The model under review builds one solid part; all positions refer to its coordinate system, in mm. A direction names the side the tool comes from. Round coordinates to 2 decimals unless told otherwise and drop trailing zeros. Loops run counter-clockwise (first coordinate to the right, second up) from the corner with the lowest first, then second, coordinate; pieces in that order, holes last. Notation, with made-up numbers: (57.25, 25.5) -> (70.25, 25.5) arc R28 ccw to (70.25, 48.5) -> close; hole circle Ø7 at (-20.75, 57.25). An arc over 180 degrees is marked (long way). Write each question's results on one line, items separated by ' | '. Start each with the question number.
Item 1: We need section D-D (x = -5). Give the boundary of the cut face in (y, z), and give its area (3 significant figures).
Item 2: Clearance check with flat-ended pins moving along their axes: pin 1 Ø7 at (x, z) = (-5, 11) entering from +Y; pin 2 Ø10.5 at (x, z) = (5, 17) entering from +Y; pin 3 Ø2.5 at (x, z) = (7, 29.5) entering from +Y. State where each tip first meets the part, or that it passes through.
Item 3: We need section C-C (x = 4.5). Give the boundary of the cut face in (y, z).
Item 4: We need section A-A (y = -15). Give the boundary of the cut face in (x, z), and give its area (3 significant figures).
Item 5: Tool access review of faces 4 (the cylindrical face through (-6.7, -21.5, 21.9)), 5 (the flat face through (0, -20.5, 22)), 6 (the flat face through (0, 25.5, 13)), 7 (the cylindrical face through (6.87, 21.49, 30.49)), 8 (the flat face through (0, -25.5, 13)): name each direction out of +Z, -Z, +X, -X, +Y, -Y from which nothing blocks a thin tool from reaching the whole face with its end or side.
Item 6: For L1, parallel to Y at x = 19, z = 3; L2, parallel to Y at x = -16.5, z = 31.5; L3, parallel to X at y = -22, z = 22, list the stretches that pass through material, from the lowest coordinate up. Write a range as from..to.
Item 7: We need section B-B (x = 19). Give the boundary of the cut face in (y, z), and give its area (3 significant figures).
Item 8: Mouldability with a two-part tool opening along X and no side actions: class faces 1 (the flat face through (-12, -21, 40)), 2 (the cylindrical face through (0.12, -21.51, 36.96)), 3 (the cylindrical face through (20.985, -21.514, 32.414)) as pulls with the +X half, pulls with the -X half, needs draft (parallel to the pull), parting line crosses it, or undercut.
from build123d import *

# Parameters (mm, degrees)
SKETCH_1_W          = 46
SKETCH_1_H          = 40
SKETCH_1_R          = 1.5
EXTRUDE_1_DEPTH     = 5
SKETCH_2_W          = 46
SKETCH_2_H          = 7.5
EXTRUDE_2_DEPTH     = 5
SKETCH_3_W          = 46
SKETCH_3_H          = 5
EXTRUDE_3_DEPTH     = 15
FILLET_1_R          = 5
FILLET_2_R          = 5
SKETCH_4_W          = 46
SKETCH_4_H          = 2
EXTRUDE_4_DEPTH     = 20
SKETCH_5_R          = 1
CUT_EXTRUDE_1_DEPTH = 2
SKETCH_6_R          = 1
CUT_EXTRUDE_2_DEPTH = 2
FILLET_3_R          = 3
FILLET_4_R          = 3
CUT_EXTRUDE_3_REACH = 70.037


with BuildPart() as part:
    # 草图1 → 凸台-拉伸1 (new body)
    with BuildSketch(Plane.XY):
        Rectangle(SKETCH_1_W, SKETCH_1_H)
        with Locations((-19, 15)):
            Circle(SKETCH_1_R, mode=Mode.SUBTRACT)
        with Locations(Location((19, 15, 0), (0, 0, 180))):
            Circle(SKETCH_1_R, mode=Mode.SUBTRACT)
        with Locations((19, -15)):
            Circle(SKETCH_1_R, mode=Mode.SUBTRACT)
        with Locations(Location((-19, -15, 0), (0, 0, 180))):
            Circle(SKETCH_1_R, mode=Mode.SUBTRACT)
    extrude(amount=EXTRUDE_1_DEPTH)

    # 草图2 → 凸台-拉伸2 (add)
    with BuildSketch(Plane.XY.offset(5)):
        with Locations((0, -23.75)):
            Rectangle(SKETCH_2_W, SKETCH_2_H)
        with Locations((0, 23.75)):
            Rectangle(SKETCH_2_W, SKETCH_2_H)
    extrude(amount=-EXTRUDE_2_DEPTH)

    # 草图3 → 凸台-拉伸3 (add)
    with BuildSketch(Plane.XY.offset(5)):
        with Locations((0, -23)):
            Rectangle(SKETCH_3_W, SKETCH_3_H)
        with Locations((0, 23)):
            Rectangle(SKETCH_3_W, SKETCH_3_H)
    extrude(amount=EXTRUDE_3_DEPTH)

    # 圆角1
    # the kernel refuses this fillet: 5 mm, written as the material it adds along each edge
    with BuildSketch(Plane(origin=(23, -25.5, 5), x_dir=(0, -1, 0), z_dir=(-1, 0, 0)), Plane(origin=(-23, 25.5, 5), x_dir=(0, 1, 0), z_dir=(1, 0, 0))) as fillet_1_piece_1:
        with BuildLine():
            CenterArc((5, 4), FILLET_1_R, 180, 53.130102354)
            Line((0, 4), (-0.1, 4))
            Line((-0.1, 4), (-0.1, 0))
            Line((-0.1, 0), (0, -0.1))
            ThreePointArc((0, -0.1), (1, -0.1), (1.94, -0.08))
            Line((1.94, -0.08), (2, 0))
        make_face()
    extrude(amount=46)

    # 圆角2
    fillet_2_edges = [part.edges().sort_by_distance(p)[0] for p in [
        (0, 27.5, 5),
        (0, -27.5, 5),
    ]]
    fillet(fillet_2_edges, radius=FILLET_2_R)

    # 草图4 → 凸台-拉伸4 (add)
    with BuildSketch(Plane.XY.offset(20)):
        with Locations((0, 21.5)):
            Rectangle(SKETCH_4_W, SKETCH_4_H)
        with Locations((0, -21.5)):
            Rectangle(SKETCH_4_W, SKETCH_4_H)
    extrude(amount=EXTRUDE_4_DEPTH)

    # 草图5 → 切除-拉伸1 (cut)
    with BuildSketch(Plane.XZ.offset(22.5)):
        with Locations((-7.5, 37.5)):
            Circle(SKETCH_5_R)
        with Locations((7.5, 37.5)):
            Circle(SKETCH_5_R)
        with Locations((-7.5, 22.5)):
            Circle(SKETCH_5_R)
        with Locations((7.5, 22.5)):
            Circle(SKETCH_5_R)
    extrude(amount=-CUT_EXTRUDE_1_DEPTH, mode=Mode.SUBTRACT)

    # 草图6 → 切除-拉伸2 (cut)
    with BuildSketch(Plane.XZ.offset(-20.5)):
        with Locations((7, 29.5)):
            Circle(SKETCH_6_R)
        with Locations(Location((-7, 29.5, 0), (0, 0, 180))):
            Circle(SKETCH_6_R)
    extrude(amount=-CUT_EXTRUDE_2_DEPTH, mode=Mode.SUBTRACT)

    # 圆角3
    # the kernel refuses this fillet: 3 mm, written as the material it adds along each edge
    with BuildSketch(Plane(origin=(-23, -22.5, 20), x_dir=(0, 0, 1), z_dir=(1, 0, 0))) as fillet_3_piece_1_section:
        with BuildLine():
            CenterArc((FILLET_3_R, FILLET_3_R), FILLET_3_R, 180, 90)
            Line((0, FILLET_3_R), (0, 0))
            Line((0, 0), (FILLET_3_R, 0))
        make_face()
    fillet_3_piece_1 = extrude(amount=46, mode=Mode.PRIVATE)
    fillet_3_piece_1 = fillet_3_piece_1 - Plane(origin=(-7.5, -23.184161647, 22.5), x_dir=(1, 0, 0), z_dir=(0, -1, 0)) * Cylinder(1, 104, mode=Mode.PRIVATE)
    fillet_3_piece_1 = fillet_3_piece_1 - Plane(origin=(7.5, -23.184161647, 22.5), x_dir=(1, 0, 0), z_dir=(0, -1, 0)) * Cylinder(1, 104, mode=Mode.PRIVATE)
    add(fillet_3_piece_1)
    with BuildSketch(Plane(origin=(23, 22.5, 20), x_dir=(0, 1, 0), z_dir=(-1, 0, 0))) as fillet_3_piece_2:
        with BuildLine():
            CenterArc((FILLET_3_R, -FILLET_3_R), FILLET_3_R, 90, 90)
            Line((0, -FILLET_3_R), (0, 0))
            Line((0, 0), (FILLET_3_R, 0))
        make_face()
    extrude(amount=46)

    # 圆角4
    fillet_4_edges = [part.edges().sort_by_distance(p)[0] for p in [
        (0, 25.5, 20),
        (0, -25.5, 20),
    ]]
    fillet(fillet_4_edges, radius=FILLET_4_R)

    # 切除-拉伸3: up to this face of the body (flat: up to its plane)
    cut_extrude_3_end = Plane(part.part.faces().sort_by_distance((0, 22.5, 31.516199688))[0])
    # 草图7 → 切除-拉伸3 (cut, up to the picked face)
    with BuildSketch(Plane.XZ.offset(22.5), mode=Mode.PRIVATE) as cut_extrude_3_sk1:
        with BuildLine():
            Line((-8, 40), (8, 40))
            ThreePointArc((8, 40), (0, 36.958405421), (-8, 40))
        make_face()
    cut_extrude_3_tool1 = split(extrude(cut_extrude_3_sk1.sketch, amount=-CUT_EXTRUDE_3_REACH, mode=Mode.PRIVATE), bisect_by=cut_extrude_3_end, keep=Keep.BOTH, mode=Mode.PRIVATE)
    # 草图7 → 切除-拉伸3 (cut, up to the picked face)
    with BuildSketch(Plane.XZ.offset(22.5), mode=Mode.PRIVATE) as cut_extrude_3_sk2:
        with BuildLine():
            Line((-23, 23), (-23, 40))
            Line((-23, 40), (-15.491933385, 40))
            ThreePointArc((-15.491933385, 40), (-21.03942095, 32.292080826), (-23, 23))
        make_face()
    cut_extrude_3_tool2 = split(extrude(cut_extrude_3_sk2.sketch, amount=-CUT_EXTRUDE_3_REACH, mode=Mode.PRIVATE), bisect_by=cut_extrude_3_end, keep=Keep.BOTH, mode=Mode.PRIVATE)
    # 草图7 → 切除-拉伸3 (cut, up to the picked face)
    with BuildSketch(Plane.XZ.offset(22.5), mode=Mode.PRIVATE) as cut_extrude_3_sk3:
        with BuildLine():
            Line((23, 23), (23, 40))
            Line((23, 40), (15.491933385, 40))
            ThreePointArc((15.491933385, 40), (21.03942095, 32.292080826), (23, 23))
        make_face()
    cut_extrude_3_tool3 = split(extrude(cut_extrude_3_sk3.sketch, amount=-CUT_EXTRUDE_3_REACH, mode=Mode.PRIVATE), bisect_by=cut_extrude_3_end, keep=Keep.BOTH, mode=Mode.PRIVATE)
    add(cut_extrude_3_tool1.solids().sort_by(Axis((0, -22.5, 38.769148), (0, 1, 0)))[0], mode=Mode.SUBTRACT)
    add(cut_extrude_3_tool2.solids().sort_by(Axis((-20.828476, -22.5, 35.901225), (0, 1, 0)))[0], mode=Mode.SUBTRACT)
    add(cut_extrude_3_tool3.solids().sort_by(Axis((20.828476, -22.5, 35.901225), (0, 1, 0)))[0], mode=Mode.SUBTRACT)


solid = part.part
Here are the results:
1) outline: (-27.5, 0) -> (27.5, 0) -> (27.5, 3) arc R5 ccw to (26.5, 6) arc R5 cw to (25.5, 9) -> (25.5, 17.8) arc R3 ccw to (24, 20.4) arc R3 cw to (22.5, 23) -> (22.5, 38.05) -> (20.5, 38.05) -> (20.5, 5) -> (-20.5, 5) -> (-20.5, 38.05) -> (-22.5, 38.05) -> (-22.5, 23) arc R3 cw to (-24, 20.4) arc R3 ccw to (-25.5, 17.8) -> (-25.5, 9) arc R5 cw to (-26.5, 6) arc R5 ccw to (-27.5, 3) -> close | area: 504 mm2
2) pin 1: stops at y = 25.73 | pin 2: stops at y = 25.5 | pin 3: stops at y = 22.5
3) outline: (-27.5, 0) -> (27.5, 0) -> (27.5, 3) arc R5 ccw to (26.5, 6) arc R5 cw to (25.5, 9) -> (25.5, 17.8) arc R3 ccw to (24, 20.4) arc R3 cw to (22.5, 23) -> (22.5, 37.83) -> (20.5, 37.83) -> (20.5, 5) -> (-20.5, 5) -> (-20.5, 37.83) -> (-22.5, 37.83) -> (-22.5, 23) arc R3 cw to (-24, 20.4) arc R3 ccw to (-25.5, 17.8) -> (-25.5, 9) arc R5 cw to (-26.5, 6) arc R5 ccw to (-27.5, 3) -> close
4) outline: (-23, 0) -> (-20.5, 0) -> (-20.5, 5) -> (-23, 5) -> close; (-17.5, 0) -> (17.5, 0) -> (17.5, 5) -> (-17.5, 5) -> close; (20.5, 0) -> (23, 0) -> (23, 5) -> (20.5, 5) -> close | area: 200 mm2
5) face 4: -Y | face 5: +Z, +X, -X | face 6: +Z, +X, -X, +Y | face 7: +Y | face 8: +Z, +X, -X, -Y
6) L1: y = -27.5..-16.5, -13.5..13.5, 16.5..27.5 | L2: y = -22.5..-20.5, 20.5..22.5 | L3: x = -23..-8.37, -6.63..6.63, 8.37..23
7) outline: (-27.5, 0) -> (-16.5, 0) -> (-16.5, 5) -> (-20.5, 5) -> (-20.5, 35.96) -> (-22.5, 35.96) -> (-22.5, 23) arc R3 cw to (-24, 20.4) arc R3 ccw to (-25.5, 17.8) -> (-25.5, 9) arc R5 cw to (-26.5, 6) arc R5 ccw to (-27.5, 3) -> close; (-13.5, 0) -> (13.5, 0) -> (13.5, 5) -> (-13.5, 5) -> close; (16.5, 0) -> (27.5, 0) -> (27.5, 3) arc R5 ccw to (26.5, 6) arc R5 cw to (25.5, 9) -> (25.5, 17.8) arc R3 ccw to (24, 20.4) arc R3 cw to (22.5, 23) -> (22.5, 35.96) -> (20.5, 35.96) -> (20.5, 5) -> (16.5, 5) -> close | area: 465 mm2
8) face 1: needs draft | face 2: undercut | face 3: pulls with the +X half
